Design review of the part shown in the three views and the two pictorial views. Dimensions are in mm from the part's minimum x, y and z. A direction names the side the tool comes from. Give positions to 0.01 mm unless a question says otherwise; leave off trailing zeros. Loops run counter-clockwise (first coordinate to the right, second up) from the corner with the lowest first, then second, coordinate; pieces in that order, holes last.
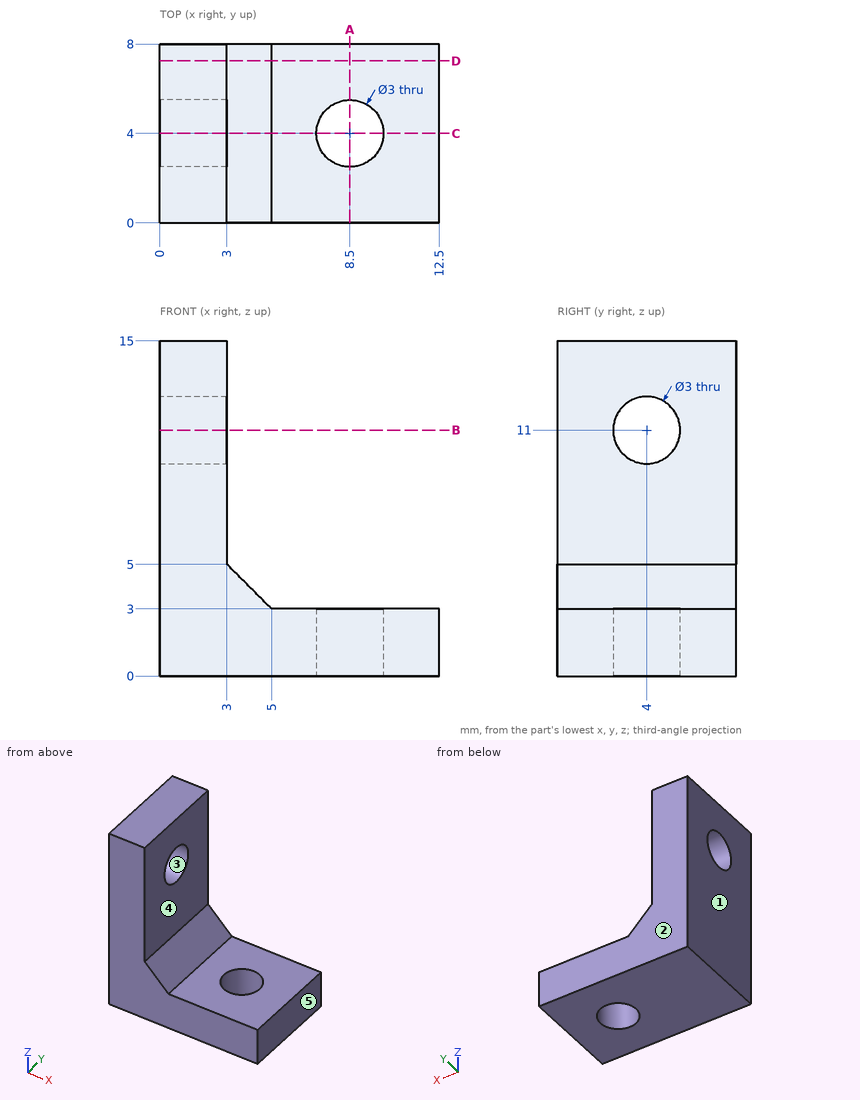
Q1. Take a section at A-A (x = 8.5). Give the boundary of the cut face in (y, z).
Results:
outline: (0, 0) - (2.5, 0) - (2.5, 3) - (0, 3) - close; (5.5, 0) - (8, 0) - (8, 3) - (5.5, 3) - close
Q2. Tool access review of the marked faces 4 and 5: name each direction out of +Z, -Z, +X, -X, +Y, -Y from which nothing blocks a thin tool from reaching the whole face with its end or side.
Results:
face 4: +Z, +X, +Y, -Y
face 5: +Z, -Z, +X, +Y, -Y
Q3. Take a section at B-B (z = 11). Give the boundary of the cut face in (x, y).
Results:
outline: (0, 0) - (3, 0) - (3, 2.5) - (0, 2.5) - close; (0, 5.5) - (3, 5.5) - (3, 8) - (0, 8) - close
Q4. Wall thickness on line 1 (X direction, y = 4, z = 1.2); line 2 (Z direction, x = 11.5, y = 4.5): over which ranges is each line inside the solid? List them lowest first.
Results:
line 1: x = 0 to 7, 10 to 12.5
line 2: z = 0 to 3
Q5. Take a section at C-C (y = 4). Give the boundary of the cut face in (x, z).
Results:
outline: (0, 0) - (7, 0) - (7, 3) - (5, 3) - (3, 5) - (3, 9.5) - (0, 9.5) - close; (0, 12.5) - (3, 12.5) - (3, 15) - (0, 15) - close; (10, 0) - (12.5, 0) - (12.5, 3) - (10, 3) - close
Q6. Take a section at D-D (y = 7.25). Give the boundary of the cut face in (x, z).
Results:
outline: (0, 0) - (12.5, 0) - (12.5, 3) - (5, 3) - (3, 5) - (3, 15) - (0, 15) - close
Q7. Insertion check: pin 1 (1.8 mm diameter, centred on y = 4, z = 11, fed in from +X); pin 2 (4 mm diameter, centred on x = 8.5, y = 3.5, fed in from +Z); pin 3 (4 mm diameter, centred on y = 2.5, z = 12, fed in from +X). Each pin has a flat end and moves straight along its axis. Give the tip position at first contact, or say it passes through.
Results:
pin 1: passes through
pin 2: stops at z = 3
pin 3: stops at x = 3
Q8. Draft analysis for pull direction Y (two halves, no side actions). For the marked faces 1, 2 and 3, state which applies: pulls with the +Y half, pulls with the -Y half, needs draft (parallel to the pull), parting line crosses it, or undercut.
Results:
face 1: needs draft
face 2: pulls with the +Y half
face 3: undercut
